Could you check a few things on this drawing? It's one solid part, dimensions in mm from its lowest x, y, z. Round coordinates to 2 decimals unless told otherwise and drop trailing zeros. Order: outer loops, then holes, each group sorted by start corner. A loop starts at its lowest first (then second) coordinate and runs counter-clockwise, first axis right, second up.
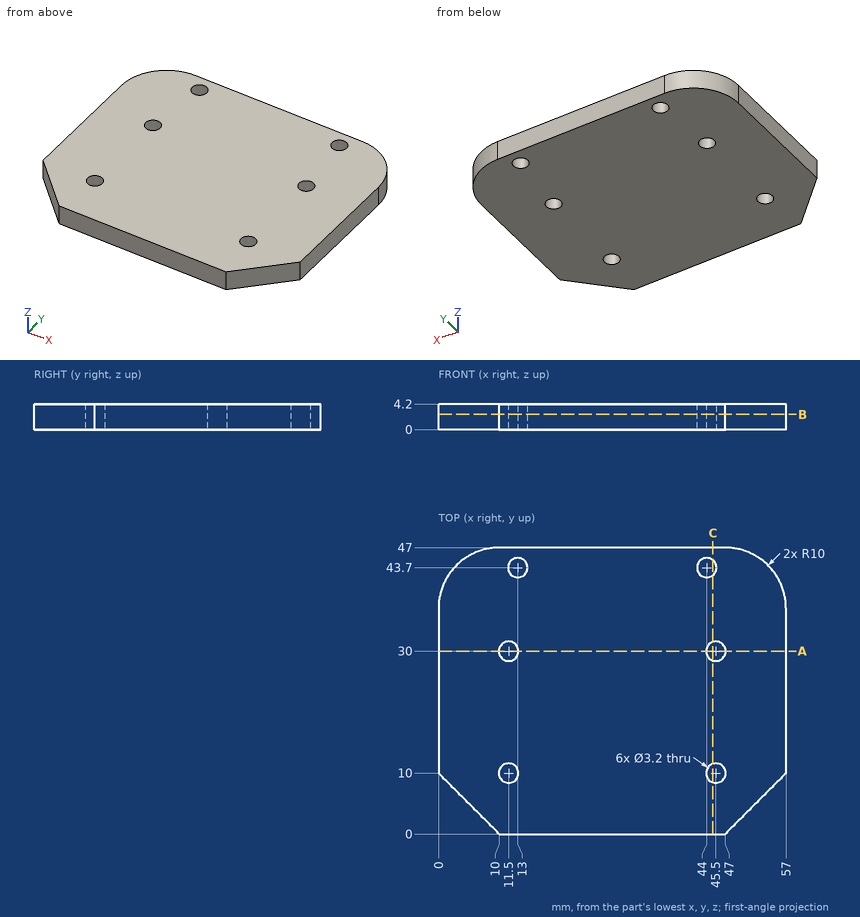
1) If we section it at B-B (z = 2.5): Write out the boundary of the cut face in (x, y), plus the area to 3 significant figures.
2) I'm going to push flat-ended pins straight in: pin 1 (2 mm diameter, centred on x = 49.5, z = 1.5, fed in from +Y); pin 2 (4 mm diameter, centred on x = 11.5, y = 30, fed in from -Z). Where does each tip first touch, or does it pass through?
3) If we section it at A-A (y = 30): Write out the boundary of the cut face in (x, z), plus the area to 3 significant figures.
4) I need wall thicknesses on line 1 (Y direction, x = 54, z = 0.9); line 2 (Y direction, x = 52, z = 0.6); line 3 (X direction, y = 8, z = 0.85). Which ranges of each line are inside material? Lowest first, please.
5) If we section it at C-C (x = 45): Write out the boundary of the cut face in (y, z).
Solutions:
1. outline: (0, 10) - (10, 0) - (47, 0) - (57, 10) - (57, 37) arc R10 ccw to (47, 47) - (10, 47) arc R10 ccw to (0, 37) - close; hole circle Ø3.2 at (11.5, 10); hole circle Ø3.2 at (11.5, 30); hole circle Ø3.2 at (13, 43.7); hole circle Ø3.2 at (44, 43.7); hole circle Ø3.2 at (45.5, 10); hole circle Ø3.2 at (45.5, 30)
1. area: 2,490 mm2
2. pin 1: stops at y = 46.89
2. pin 2: stops at z = 0
3. outline: (0, 0) - (9.9, 0) - (9.9, 4.2) - (0, 4.2) - close; (13.1, 0) - (43.9, 0) - (43.9, 4.2) - (13.1, 4.2) - close; (47.1, 0) - (57, 0) - (57, 4.2) - (47.1, 4.2) - close
3. area: 213 mm2
4. line 1: y = 7 to 44.14
4. line 2: y = 5 to 45.66
4. line 3: x = 2 to 55
5. outline: (0, 0) - (8.48, 0) - (8.48, 4.2) - (0, 4.2) - close; (11.52, 0) - (28.48, 0) - (28.48, 4.2) - (11.52, 4.2) - close; (31.52, 0) - (42.45, 0) - (42.45, 4.2) - (31.52, 4.2) - close; (44.95, 0) - (47, 0) - (47, 4.2) - (44.95, 4.2) - close
